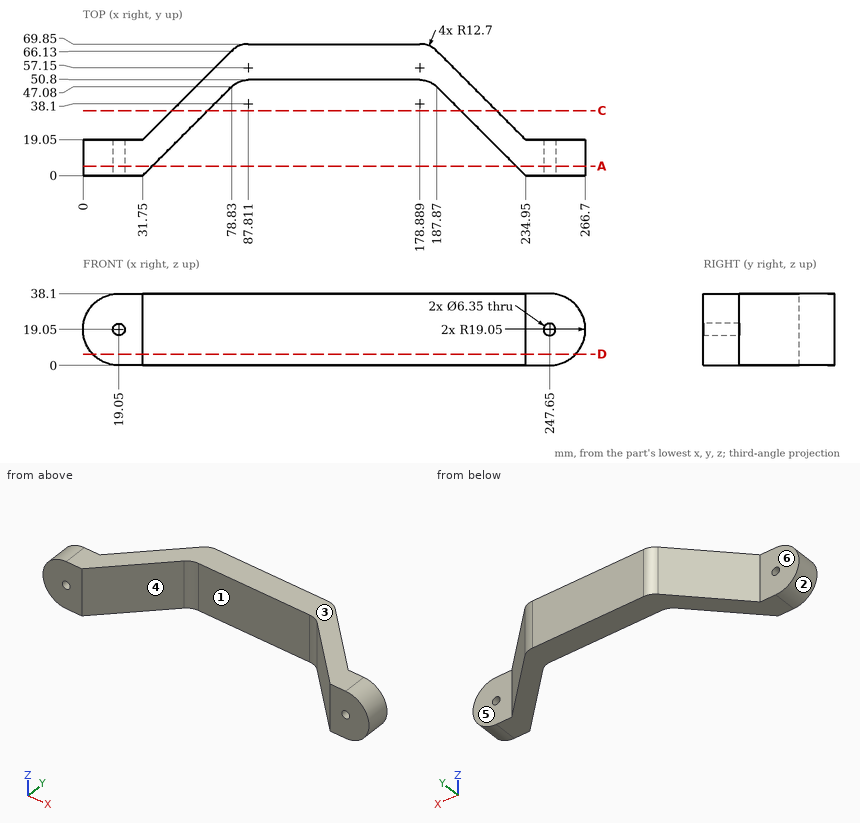
Can you work these out from the drawing? Everything is in mm from the part's minimum corner. A direction names the side the tool comes from. Round coordinates to 2 decimals unless told otherwise and drop trailing zeros. Order: outer loops, then holes, each group sorted by start corner. A loop starts at its lowest first (then second) coordinate and runs counter-clockwise, first axis right, second up.
(1) If we section it at D-D (z = 6): Please give me the cut outline in (x, y), plus the area to 3 significant figures.
Results are:
outline: (5.17, 0) - (31.75, 0) - (78.83, 47.08) arc R12.7 cw to (87.81, 50.8) - (178.89, 50.8) arc R12.7 cw to (187.87, 47.08) - (234.95, 0) - (261.53, 0) - (261.53, 19.05) - (234.95, 19.05) - (187.87, 66.13) arc R12.7 ccw to (178.89, 69.85) - (87.81, 69.85) arc R12.7 ccw to (78.83, 66.13) - (31.75, 19.05) - (5.17, 19.05) - close
area: 4,880 mm2
(2) If I drill on L1, parallel to Z at x = 247.65, y = 15 (1 decimal); L2, parallel to Y at x = 95.5, z = 10; L3, parallel to X at y = 7.75, z = 19.05 (1 decimal), over which ranges is the centre line in solid material (lowest first)?
Results are:
L1: z = 0 to 15.9, 22.2 to 38.1
L2: y = 50.8 to 69.85
L3: x = 0 to 15.9, 22.2 to 39.5, 227.2 to 244.5, 250.8 to 266.7
(3) If we section it at C-C (y = 34.5): Please give me the cut outline in (x, z), plus the area to 3 significant figures.
Results are:
outline: (47.2, 0) - (66.25, 0) - (66.25, 38.1) - (47.2, 38.1) - close; (200.45, 0) - (219.5, 0) - (219.5, 38.1) - (200.45, 38.1) - close
area: 1,450 mm2
(4) On a 3-axis mill with a long thin cutter (end or side, diameter ignored), from which of +Z, -Z, +X, -X, +Y, -Y can I reach the whole of each face in a straight line? I mean the marked faces 4, 5 and 6. Say none if no direction works.
Results are:
face 4: +Z, -Z, -Y
face 5: +Z, -Z, +X, +Y
face 6: +Z, -Z, -X, +Y
(5) I'm going to push flat-ended pins straight in: pin 1 (16 mm diameter, centred on x = 250, z = 25.5, fed in from +Y); pin 2 (10 mm diameter, centred on x = 211, y = 23, fed in from -Z); pin 3 (6 mm diameter, centred on y = 17, z = 21.5, fed in from -X); pin 4 (6 mm diameter, centred on x = 211, z = 26.5, fed in from +Y). Where does each tip first touch, or does it pass through?
Results are:
pin 1: stops at y = 19.05
pin 2: stops at z = 0
pin 3: stops at x = 0
pin 4: stops at y = 46
(6) We'd pull the mould along X, two halves only. Please class the marked faces 1, 2 and 3: +X half, -X half, draft (parallel to the pull), parting line (faces both ways), or undercut.
Results are:
face 1: undercut
face 2: -X half
face 3: draft
(7) If we section it at A-A (y = 5): Count the separate pieces of the cut face and the enclosed holes in it, plus the area to 3 significant figures.
Results are:
separate pieces: 2
enclosed holes: 2
area: 2,430 mm2
